Autodesk Inventor part; units mm, degrees
ref_plane "Work Plane1" through (66.6877, 0, 0) normal (0, 0, -1) x (1, 0, 0)
ref_plane "YZ Plane" through (0, 0, 0) normal (1, 0, 0) x (0, 1, 0)
ref_plane "XZ Plane" through (0, 0, 0) normal (0, 1, 0) x (-1, 0, 0)
sketch "Sketch1" plane through (0, 0, 0) normal (0, 0, 1) x (1, 0, 0)
  line L0 (22.225, 0) -> (22.225, 1.7526)
  line L1 (22.225, 1.7526) -> (2.4638, 1.7526)
  line L2 (0, 3.3401) -> (0, 1.2192)
  line L3 (0, 1.2192) -> (1.6764, 1.2192)
  line L4 (1.6764, 1.2192) -> (2.3803, 0)
  line L5 (2.3803, 0) -> (22.225, 0)
  line L6 (0, 3.3401) -> (0.6376, 3.3401)
  line L7 (0.6376, 3.3401) -> (2.4638, 1.7526)
  line L8 (-4.445, 0) -> (26.67, 0)
  line L9 (0, -0.668) -> (0, 4.0081)
  dimension "d0" = 22.225
  dimension "d1" = 1.6764
  dimension "d2" = 3.5052
  dimension "d3" = 2.4638
  dimension "d4" = 41
  dimension "d5" = 2.4384
  dimension "d6" = 60
  dimension "d7" = 6.6802
revolve "Body" add sketch "Sketch1" angle 360 about axis through (2.3803, 0, 0) along (1, 0, 0) contours L5 L4 L3 L2 L6 L7 L1 L0
sketch "Sketch2" plane through (0, 0, 0) normal (-1, 0, 0) x (0, 0, 1)
  circle A0 centre (0, 0) radius 3.3401
  circle A1 centre (0, 0) radius 1.2192
  line L0 (0.9421, 0.2524) -> (1.1777, 0.3156)
  line L1 (0.9421, -0.2524) -> (1.1777, -0.3156)
  arc A2 (0.9421, -0.2524) -> (0.9421, 0.2524) centre (0, 0) ccw
  arc A3 (1.1777, -0.3156) -> (1.1777, 0.3156) centre (0, 0) ccw
  line L2 (0, -4.6761) -> (0, 4.6761)
  line L3 (-4.6761, 0) -> (4.6761, 0)
  line L4 (0.9421, 0.2524) -> (0, 0) construction
  line L5 (0, 0) -> (0.9421, -0.2524) construction
  line L6 (0.2524, 0.9421) -> (0.3156, 1.1777)
  line L7 (0.6897, 0.6897) -> (0.8621, 0.8621)
  arc A4 (0.6897, 0.6897) -> (0.2524, 0.9421) centre (0, 0) ccw
  arc A5 (0.8621, 0.8621) -> (0.3156, 1.1777) centre (0, 0) ccw
  line L8 (-0.6897, 0.6897) -> (-0.8621, 0.8621)
  line L9 (-0.2524, 0.9421) -> (-0.3156, 1.1777)
  arc A6 (-0.2524, 0.9421) -> (-0.6897, 0.6897) centre (0, 0) ccw
  arc A7 (-0.3156, 1.1777) -> (-0.8621, 0.8621) centre (0, 0) ccw
  line L10 (-0.9421, -0.2524) -> (-1.1777, -0.3156)
  line L11 (-0.9421, 0.2524) -> (-1.1777, 0.3156)
  arc A8 (-0.9421, 0.2524) -> (-0.9421, -0.2524) centre (0, 0) ccw
  arc A9 (-1.1777, 0.3156) -> (-1.1777, -0.3156) centre (0, 0) ccw
  line L12 (-0.2524, -0.9421) -> (-0.3156, -1.1777)
  line L13 (-0.6897, -0.6897) -> (-0.8621, -0.8621)
  arc A10 (-0.6897, -0.6897) -> (-0.2524, -0.9421) centre (0, 0) ccw
  arc A11 (-0.8621, -0.8621) -> (-0.3156, -1.1777) centre (0, 0) ccw
  line L14 (0.6897, -0.6897) -> (0.8621, -0.8621)
  line L15 (0.2524, -0.9421) -> (0.3156, -1.1777)
  arc A12 (0.2524, -0.9421) -> (0.6897, -0.6897) centre (0, 0) ccw
  arc A13 (0.3156, -1.1777) -> (0.8621, -0.8621) centre (0, 0) ccw
  dimension "d8" = 1.9507
  dimension "d9" = 2.4384
  dimension "d10" = 15
  dimension "d11" = 15
  dimension "d22" = 360
extrude "Slot" add sketch "Sketch2" against normal up to next contours L3 A2 L0 A1 | A1 L1 A2 L3 | L3 A8 L10 A1 | A1 L11 A8 L3 | A1 L7 A4 L6 | L9 A6 L8 A1 | A1 L13 A10 L12 | L15 A12 L14 A1
thread "Thread"
chamfer "Chamfer1" distance 0.4724 distance2 0.9449 1 edges at (22.225, -1.7526, 0) measured on face at (22.225, -0.4543, 0.2476)
ref_plane "Work Plane1" through (66.6877, 0, 0) normal (0, 0, -1) x (1, 0, 0)
equation "\"d0\" = NLG"
equation "\"d1\" = INTI"
equation "\"d2\" = GD"
equation "\"d3\" = KOH"
equation "\"d4\" = 0.5 * SEWI"
equation "\"d5\" = SW"
equation "\"d7\" = KOD"
equation "\"d8\" = 0.8 * SW"
equation "\"d9\" = SW"
equation "\"d15\" = GEL"
equation "\"d17\" = -0.5 * SPD + 0.5 * GD"
equation "\"d18\" = GUL"
equation "\"NLG\" = 22.225"
equation "\"SW\" = 2.4384"
equation "\"INTI\" = 1.6764"
equation "\"GEL\" = 17.77695"
equation "\"KOH\" = 2.4638"
equation "\"KOD\" = 6.6802"
equation "\"GUL\" = 0.94488"
equation "\"SPD\" = 2.56032"
equation "\"GD\" = NND"
equation "\"SEWI\" = 82deg"
equation "\"TOA\" = 30deg"
equation "\"GD1\" = SPD"
equation "\"EPV\" = 4.4794"
equation "\"THREADDIA\" = 3.5052"
equation "\"BDM\" = NND"
equation "\"NND\" = 3.5052"
equation "\"GAL\" = 1.9845"
equation "\"E0\" = 1.155 * SW"
properties part number "ANSI B18.3 - 6-32 UNC x 0.875, SSFCHCSI" material "Steel, Mild"
Input: part model. Units: mm. Frame: model coordinates. A direction names the side the tool comes from. Coordinates: 2 decimals unless noted, no trailing zeros. Order: outer loops, then holes, each group sorted by start corner. A loop starts at its lowest first (then second) coordinate and runs counter-clockwise, first axis right, second up. Notation, with made-up numbers: M 5,-38 L 40,-38 A21 cw 40,-5 Z; hole C -25,-20 d1. An arc over 180 degrees is marked long. Answer as CSV lines item,"result".
1. Access query for faces 4 (the cylindrical face through (11.74, 1.67, -0.53)), 5 (the flat face through (0, -1, -1)). Directions: +Z, -Z, +X, -X, +Y, -Y. A direction counts if a zero-diameter tool reaches every point of the face in a straight line with its end or side. Return the directions, or none.
Reported:
face 4,"+X"
face 5,"+Z, -Z, -X, +Y, -Y"
2. Pull-direction query (Y, two-part tool) for faces 1 (the cylindrical face through (0.323, 1.796, 2.816)), 2 (the conical face through (2.34, -0.02, 0.07)), 3 (the flat face through (22.225, 0, 0)); classes: released by +Y, released by -Y, zero draft, split by the parting line, or undercut.
Reported:
face 1,"split by the parting line"
face 2,"undercut"
face 3,"zero draft"
3. Material intervals for line 1 (Z direction, x = 1.5, y = 0.5); line 2 (X direction, y = -1.75, z = 0.75); line 3 (Z direction, x = 16, y = 1.25), sorted ascending. Write a range as from..to.
Reported:
line 1,"-2.54..-1.11, 1.11..2.54"
line 2,"0..2.29"
line 3,"-1.23..1.23"
4. First-contact query: P1, Ø1.5, axis at x = 17, y = 1.5, coming from the +Z side; P2, Ø1.5, axis at x = 15, y = 0.5, coming from the +Z side; P3, Ø1.5, axis at x = 8, z = 2, coming from the -Y side. Flat tips, straight axial feed; report the tip coordinate or a pass-through.
Reported:
P1,"z = 1.58"
P2,"z = 1.75"
P3,"y = -1.23"
5. Section A-A (x = 6.5). Return the cut outline in (y, z).
Reported:
outline,"C 0,0 d3.51"
